from build123d import *

# Parameters (mm, degrees)
F0_W     = 25
F0_H     = 2
F1_DEPTH = 5
F2_R     = 1
F3_R     = 1


with BuildPart() as f1:
    # F0 (on Top) → F1 (new body)
    with BuildSketch(Plane.XY):
        with BuildLine():
            Line((-26.404906, 10.2), (-25, 10.2))
            Line((-25, 10.2), (-23, 10.2))
            add(Edge.make_bspline(
                [(-23, 10.2), (-23.017775, 11.829905), (-23.894977, 11.75835), (-25.660651, 11.815999)],
                knots=[0, 0, 0, 0, 3.112959, 3.112959, 3.112959, 3.112959], degree=3))
            Line((-25.660651, 11.815999), (-26.404906, 10.2))
        make_face()
        Polygon((-27, 0), (-25, 0), (-25, 2), (-25, 10.2), (-26.404906, 10.2), align=None)
        with Locations((-12.5, 1)):
            Rectangle(F0_W, F0_H)
        with Locations((12.5, 1)):
            Rectangle(F0_W, F0_H)
        Polygon((25, 2), (25, 0), (27, 0), (26.404906, 10.2), (25, 10.2), align=None)
        with BuildLine():
            Line((23, 10.2), (25, 10.2))
            Line((25, 10.2), (26.404906, 10.2))
            Line((26.404906, 10.2), (25.660651, 11.815999))
            add(Edge.make_bspline(
                [(23, 10.2), (23.017775, 11.829905), (23.894977, 11.75835), (25.660651, 11.815999)],
                knots=[0, 0, 0, 0, 3.112959, 3.112959, 3.112959, 3.112959], degree=3))
        make_face()
    extrude(amount=F1_DEPTH)

    # F2
    f2_edges = [f1.edges().sort_by_distance(p)[0] for p in [
        (25.660651, 11.815999, 2.5),
    ]]
    fillet(f2_edges, radius=F2_R)

    # F3
    f3_edges = [f1.edges().sort_by_distance(p)[0] for p in [
        (-25.660651, 11.815999, 2.5),
    ]]
    fillet(f3_edges, radius=F3_R)


solid = f1.part
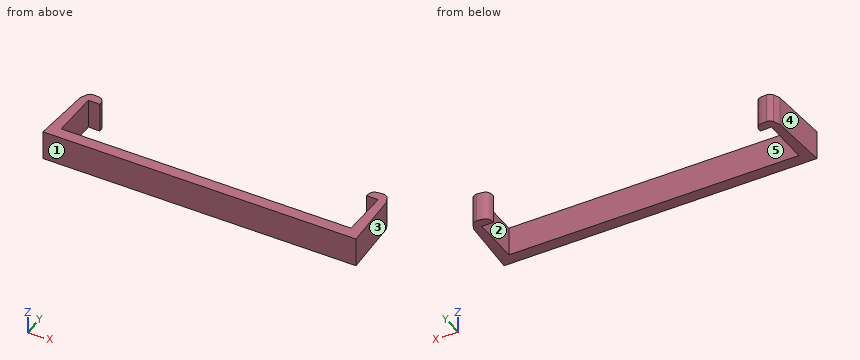
Read the model definition and answer for the solid it produces. Units are mm, in the model's axes. Face numbers are marked on the shaded views. A direction names the side the tool comes from. Give positions to 0.01 mm unless a question says otherwise; leave off trailing zeros. Write each loop counter-clockwise with the first axis right and the second up, starting at its lowest first coordinate (ties: lowest second). Pieces come first, ordered by that corner, then holes. Notation, with made-up numbers: (80.25, -21) - (86.25, -21) arc R29 ccw to (86.25, 1) - close; hole circle Ø9 at (87, 74). An arc over 180 degrees is marked (long way). Use CSV: the item, a comma, the result in double quotes. Start each with the question number.
(1) Find section C-C (x = 9). Give the vertices of the cut face in (y, z).
(2) Find section B-B (y = 9.75). Give the vertices of the cut face in (x, z).
(3) Find section A-A (y = 5.25). Give the vertices of the cut face in (x, z), plus the area to 3 significant figures.
(4) Given P1, Ø1.5, axis at y = 8, z = 3.5, coming from the -X side; P2, Ø2, axis at x = -24.5, z = 1.5, coming from the -Y side; P3, Ø1, axis at y = 7, z = 3.5, coming from the +X side; P4, Ø1.5, axis at y = 6, z = 2, coming from the +X side, each flat-ended and moving along its own axis, determine where each tip first touches the part or whether it passes through.
(5) For the marked faces 1 and 2, determine the directions among +Z, -Z, +X, -X, +Y, -Y from which every point of the face is accessible in a straight line to the end or side of a thin tool.
(6) Consider line 1 along X through (y, z) = (10, 1.2); line 2 along Y through (x, z) = (-5, 0.3); line 3 along X through (y, z) = (4, 4.6). Determine where each line is inside the solid, lowest interval first.
(7) Determine the mould class of the marked faces 3, 4 and 5 for opening direction X: +X half, -X half, draft (parallel to the pull), parting line (faces both ways), or undercut.
Findings below:
1,outline,"(0, 0) - (2, 0) - (2, 5) - (0, 5) - close"
2,outline,"(-26.43, 0) - (-25, 0) - (-25, 5) - (-26.43, 5) - close; (25, 0) - (26.43, 0) - (26.43, 5) - (25, 5) - close"
3,outline,"(-26.69, 0) - (-25, 0) - (-25, 5) - (-26.69, 5) - close; (25, 0) - (26.69, 0) - (26.69, 5) - (25, 5) - close"
3,area,"16.9 mm2"
4,P1,"x = -26.58"
4,P2,"y = 0"
4,P3,"x = 26.62"
4,P4,"x = 26.69"
5,face 1,"+Z, -Z, +X, -X, -Y"
5,face 2,"+Z, -Z"
6,line 1,"-26.42 to -25, 25 to 26.42"
6,line 2,"0 to 2"
6,line 3,"-26.77 to -25, 25 to 26.77"
7,face 3,"+X half"
7,face 4,"-X half"
7,face 5,"undercut"
